Verification items for the finished model (mm, model axes). A direction names the side the tool comes from. Round coordinates to 2 decimals unless told otherwise and drop trailing zeros. Write each loop counter-clockwise with the first axis right and the second up, starting at its lowest first coordinate (ties: lowest second). Pieces come first, ordered by that corner, then holes. Notation, with made-up numbers: (70.5, -13) - (90.5, -13) arc R15 ccw to (90.5, 6) - close; hole circle Ø6 at (-17, 17). An arc over 180 degrees is marked (long way). Answer as a JSON object with one key per item and string values. Group by question number.
1) Section check D-D (y = 10.5). Enter the section's corners in (x, z).
2) Go/stop test with flat-tipped pins: pin 1 Ø2.5 at (x, y) = (15, 0) entering from +Z; pin 2 Ø0.8 at (x, z) = (6, 0.5) entering from +Y. Record where each tip stops, or that it passes through.
3) Section check B-B (y = 0). Enter the section's corners in (x, z).
4) Section check A-A (x = 15). Enter the section's corners in (y, z).
5) Section check C-C (z = 0.65). Enter the section's corners in (x, y).
6) Mould release check, pull along X, two halves, no side actions. Record for faces 1 (the flat face through (-37.85, 5.02, 0.49)), 2 (the flat face through (-28, 1, 1)), 3 (the flat face through (-36.04, 8.87, 0.49)), 4 (the cylindrical face through (-89.15, -11.9, 0.49)): +X half, -X half, draft (parallel to the pull), parting line (faces both ways), or undercut.
7) Set-up check for faces 5 (the cylindrical face through (29, 0, 1.5)), 6 (the flat face through (-65.16, -0.3, 0.49)), 7 (the flat face through (-28.4, 1.7, 0)): record each of +Z, -Z, +X, -X, +Y, -Y from which the full face is reachable in a straight line by a thin tool's end or side.
8) Thickness scan on line 1 (Y direction, x = 15, z = 0.25); line 2 (Y direction, x = -23, z = 0.85); line 3 (X direction, y = -6, z = 0.75). Record the ranges inside material, lowest first.
```python
from build123d import *

# Parameters (mm, degrees)
SKETCH_1_R      = 1
EXTRUDE_1_DEPTH = 1
SKETCH_2_R      = 1
EXTRUDE_2_DEPTH = 1


with BuildPart() as part:
    # 草图1 → 凸台-拉伸1 (new body)
    with BuildSketch(Plane.XY):
        with BuildLine():
            Line((0, 2), (30, 2))
            ThreePointArc((30, 2), (32, 0), (30, -2))
            Line((30, -2), (0, -2))
            Line((0, -2), (-30, -2))
            ThreePointArc((-30, -2), (-30.765366865, -1.847759065), (-31.414213562, -1.414213562))
            Line((-31.414213562, -1.414213562), (-44.471184953, 11.642757828))
            Line((-44.471184953, 11.642757828), (-86.443405813, -12.589915184))
            ThreePointArc((-86.443405813, -12.589915184), (-89.175456621, -11.857864376), (-88.443405813, -9.125813569))
            Line((-88.443405813, -9.125813569), (-45.142135624, 15.874186431))
            ThreePointArc((-45.142135624, 15.874186431), (-43.881083239, 16.125025346), (-42.727922061, 15.556349186))
            Line((-42.727922061, 15.556349186), (-29.171572875, 2))
            Line((-29.171572875, 2), (0, 2))
        make_face()
        with Locations((15, 0)):
            Circle(SKETCH_1_R, mode=Mode.SUBTRACT)
        Circle(SKETCH_1_R, mode=Mode.SUBTRACT)
    extrude(amount=EXTRUDE_1_DEPTH)

    # 草图2 → 凸台-拉伸2 (add)
    with BuildSketch(Plane.XY.offset(1)):
        with Locations((30, 0)):
            Circle(SKETCH_2_R)
    extrude(amount=EXTRUDE_2_DEPTH)


solid = part.part
```
Returned:
{
 "1": {"outline": "(-54.45, 0) - (-46.45, 0) - (-46.45, 1) - (-54.45, 1) - close; (-43.33, 0) - (-37.67, 0) - (-37.67, 1) - (-43.33, 1) - close"},
 "2": {"pin 1": "z = 1", "pin 2": "y = 2"},
 "3": {"outline": "(-72.64, 0) - (-64.64, 0) - (-64.64, 1) - (-72.64, 1) - close; (-32.83, 0) - (-1, 0) - (-1, 1) - (-32.83, 1) - close; (1, 0) - (14, 0) - (14, 1) - (1, 1) - close; (16, 0) - (32, 0) - (32, 1) - (31, 1) - (31, 2) - (29, 2) - (29, 1) - (16, 1) - close"},
 "4": {"outline": "(-2, 0) - (-1, 0) - (-1, 1) - (-2, 1) - close; (1, 0) - (2, 0) - (2, 1) - (1, 1) - close"},
 "5": {"outline": "(-88.44, -9.13) arc R2 ccw to (-86.44, -12.59) - (-44.47, 11.64) - (-31.41, -1.41) arc R2 ccw to (-30, -2) - (30, -2) arc R2 ccw to (30, 2) - (-29.17, 2) - (-42.73, 15.56) arc R2 ccw to (-45.14, 15.87) - close; hole circle Ø2 at (0, 0); hole circle Ø2 at (15, 0)"},
 "6": {"face 1": "undercut", "face 2": "draft", "face 3": "+X half", "face 4": "parting line"},
 "7": {"face 5": "+Z", "face 6": "+Z, -Z, -Y", "face 7": "-Z, +X, -X, +Y, -Y"},
 "8": {"line 1": "-2 to -1, 1 to 2", "line 2": "-2 to 2", "line 3": "-83.03 to -75.03"}
}
